```python
from build123d import *

# Parameters (mm, degrees)
SKETCH1_R            = 12.7
BOSS_EXTRUDE1_DEPTH  = 22.86
SKETCH2_R            = 6.35
BOSS_EXTRUDE2_DEPTH  = 3.81
SKETCH4_W            = 41.167859691
SKETCH4_H            = 25.4
BOSS_EXTRUDE4_DEPTH  = 4.318
FILLET3_R            = 2.380000066
FILLET4_R            = 10
SKETCH5_W            = 10.234607526
SKETCH5_H            = 25.4
BOSS_EXTRUDE5_DEPTH  = 20.32
SKETCH8_W            = 41.167859691
SKETCH8_H            = 25.4
BOSS_EXTRUDE10_DEPTH = 4.318
FILLET12_R           = 4.92
FILLET13_R           = 4.92
SKETCH9_R            = 5.08
CUT_EXTRUDE1_DEPTH   = 1.524
CUT_EXTRUDE3_START   = 1.524
SKETCH10_R           = 5.08
CUT_EXTRUDE3_DEPTH   = 1.524


with BuildPart() as part:
    # Sketch1 → Boss-Extrude1 (new body)
    with BuildSketch(Plane(origin=(0, 0, 0), x_dir=(0, 0, -1), z_dir=(1, 0, 0))):
        Circle(SKETCH1_R)
    extrude(amount=BOSS_EXTRUDE1_DEPTH)

    # Sketch2 → Boss-Extrude2 (add)
    with BuildSketch(Plane(origin=(22.86, 0, 0), x_dir=(0, 0, -1), z_dir=(1, 0, 0))):
        with Locations(Location((0, 0, 0), (0, 0, 180))):
            Circle(SKETCH2_R)
    extrude(amount=BOSS_EXTRUDE2_DEPTH)

    # Sketch4 → Boss-Extrude4 (add)
    with BuildSketch(Plane.XY.offset(10.16)):
        with Locations((-20.583929846, 0)):
            Rectangle(SKETCH4_W, SKETCH4_H)
    extrude(amount=BOSS_EXTRUDE4_DEPTH)

    # Fillet3
    fillet3_edges = [part.edges().sort_by_distance(p)[0] for p in [
        (-20.583929846, 12.7, 14.478),
    ]]
    fillet(fillet3_edges, radius=FILLET3_R)

    # Fillet4
    # the kernel refuses this fillet: 10 mm, written as the material it takes off along each edge
    with BuildSketch(Plane(origin=(-61.740121963, -12.7, 14.478), x_dir=(0, 1, 0), z_dir=(1, 0, 0))) as fillet4_piece_1:
        with BuildLine():
            CenterArc((8.228904909, -10), FILLET4_R, 90, 55.375198577)
            Line((0, -4.318), (-0.164578098, -4.20436))
            ThreePointArc((-0.164578098, -4.20436), (-0.2, -2.159), (-0.2, 0))
            Line((-0.2, 0), (0, 0.2))
            Line((0, 0.2), (8.228904909, 0.2))
            Line((8.228904909, 0.2), (8.228904909, 0))
        make_face()
    extrude(amount=82.312384236, mode=Mode.SUBTRACT)

    # Sketch5 → Boss-Extrude5 (add)
    with BuildSketch(Plane.XY.offset(10.16)):
        with Locations((-5.117303763, 0)):
            Rectangle(SKETCH5_W, SKETCH5_H)
    extrude(amount=-BOSS_EXTRUDE5_DEPTH)

    # Sketch8 → Boss-Extrude10 (add)
    with BuildSketch(Plane.XY.offset(-10.16)):
        with Locations((-20.583929846, 0)):
            Rectangle(SKETCH8_W, SKETCH8_H)
    extrude(amount=-BOSS_EXTRUDE10_DEPTH)

    # Fillet12
    fillet12_edges = [part.edges().sort_by_distance(p)[0] for p in [
        (-20.583929846, 12.7, -14.478),
    ]]
    fillet(fillet12_edges, radius=FILLET12_R)

    # Fillet13
    fillet13_edges = [part.edges().sort_by_distance(p)[0] for p in [
        (-20.583929846, -12.7, -14.478),
    ]]
    fillet(fillet13_edges, radius=FILLET13_R)

    # Sketch9 → Cut-Extrude1 (cut)
    with BuildSketch(Plane.XY.offset(-10.16)):
        with Locations((-34.29, 0)):
            Circle(SKETCH9_R)
    extrude(amount=-CUT_EXTRUDE1_DEPTH, mode=Mode.SUBTRACT)

    # Sketch10 → Cut-Extrude3 (cut)
    with BuildSketch(Plane.XY.offset(10.16).offset(CUT_EXTRUDE3_START)):
        with Locations((-34.29, 0)):
            Circle(SKETCH10_R)
    extrude(amount=-CUT_EXTRUDE3_DEPTH, mode=Mode.SUBTRACT)


solid = part.part
```
For this review, take the finished solid that the model builds, in its own axes (mm). A direction names the side the tool comes from. Round coordinates to 2 decimals unless told otherwise and drop trailing zeros. Write each loop counter-clockwise with the first axis right and the second up, starting at its lowest first coordinate (ties: lowest second). Pieces come first, ordered by that corner, then holes. Notation, with made-up numbers: (29, 3.25) -> (45, 3.25) arc R19 ccw to (45, 26.25) -> close; hole circle Ø11 at (-39, 0.5). An arc over 180 degrees is marked (long way). One line per question, with ' | ' between items. Start each with the question number.
1) Mouldability with a two-part tool opening along X and no side actions: class faces 4 (the flat face through (22.86, 6, -3)), 5 (the flat face through (-34, 0, 11.684)), 6 (the cylindrical face through (-20.296, -11.297, -12.999)), 7 (the cylindrical face through (-39.365, 0.223, 10.933)) as +X half, -X half, draft (parallel to the pull), parting line (faces both ways), or undercut.
2) Add section C-C (z = 8). Write out the cut boundary in (x, y), and give its area (3 significant figures).
3) Add section D-D (x = 21). Write out the cut boundary in (y, z), and give its area (3 significant figures).
4) Machinability: for faces 1 (the cylindrical face through (24.738, 5.634, 2.93)), 2 (the flat face through (0, 1, -13)), 3 (the flat face through (-26, 0, 10.16)), which of the approach directions +Z, -Z, +X, -X, +Y, -Y give a long, thin tool a straight path to every point of the face, cutting with its end or side? Answer none if there is none.
5) For pin 1 Ø4 at (y, z) = (3.5, 11.5) entering from +X; pin 2 Ø2 at (x, z) = (6, -2.5) entering from -Y, all flat-tipped, find the tip position at first contact; note any pin that passes through.
6) Add section A-A (x = -34.29). Write out the cut boundary in (y, z), and give its area (3 significant figures).
7) Add section B-B (y = 0). Write out the cut boundary in (x, z), and give its area (3 significant figures).
8) Wall thickness on line 1 along Z through (x, y) = (-33.5, -2); line 2 along X through (y, z) = (7.75, -13.5); line 3 along X through (y, z) = (-7.75, 3.75): over which ranges is each line inside the solid? List them lowest first.
Reported:
1) face 4: +X half | face 5: undercut | face 6: draft | face 7: undercut
2) outline: (-10.23, -12.7) -> (0, -12.7) -> (0, -9.86) -> (22.86, -9.86) -> (22.86, 9.86) -> (0, 9.86) -> (0, 12.7) -> (-10.23, 12.7) -> close | area: 711 mm²
3) outline: circle Ø25.4 at (0, 0) | area: 507 mm²
4) face 1: +X | face 2: -Z, +X | face 3: -X, +Y, -Y
5) pin 1: stops at x = 22.86 | pin 2: stops at y = -12.61
6) outline: (-12.7, 10.16) -> (-5.08, 10.16) -> (-5.08, 11.68) -> (5.08, 11.68) -> (5.08, 10.16) -> (12.7, 10.16) -> (12.7, 12.1) arc R2.38 ccw to (10.32, 14.48) -> (-4.47, 14.48) arc R10 ccw to start; (-12.66, -10.16) arc R4.92 ccw to (-7.78, -14.48) -> (7.78, -14.48) arc R4.92 ccw to (12.66, -10.16) -> (5.08, -10.16) -> (5.08, -11.68) -> (-5.08, -11.68) -> (-5.08, -10.16) -> close | area: 166 mm²
7) outline: (-41.17, -14.48) -> (0, -14.48) -> (0, -12.7) -> (22.86, -12.7) -> (22.86, -6.35) -> (26.67, -6.35) -> (26.67, 6.35) -> (22.86, 6.35) -> (22.86, 12.7) -> (0, 12.7) -> (0, 14.48) -> (-41.17, 14.48) -> (-41.17, 10.16) -> (-39.37, 10.16) -> (-39.37, 11.68) -> (-29.21, 11.68) -> (-29.21, 10.16) -> (-10.23, 10.16) -> (-10.23, -10.16) -> (-29.21, -10.16) -> (-29.21, -11.68) -> (-39.37, -11.68) -> (-39.37, -10.16) -> (-41.17, -10.16) -> close | area: 1,160 mm²
8) line 1: z = -14.48 to -11.68, 11.68 to 14.48 | line 2: x = -41.17 to 0 | line 3: x = -10.23 to 22.86
